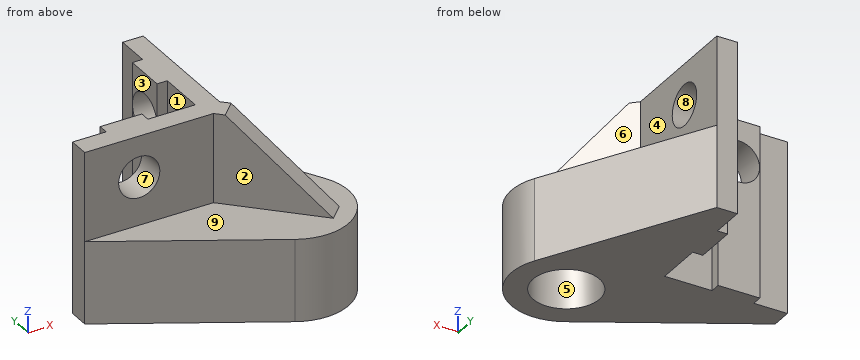
from build123d import *

# Parameters (mm, degrees)
BOSS_EXTRUDE1_DEPTH = 25
SKETCH2_R           = 3
CUT_EXTRUDE1_DEPTH  = 15
SKETCH3_R           = 3
CUT_EXTRUDE2_DEPTH  = 15
BOSS_EXTRUDE2_DEPTH = 12
BOSS_EXTRUDE4_DEPTH = 1.5
SKETCH6_R           = 4.85
CUT_EXTRUDE3_DEPTH  = 9


with BuildPart() as part:
    # Sketch1 → Boss-Extrude1 (new body)
    with BuildSketch(Plane.XY):
        Polygon((227.088719843, 62.282971172), (227.088719843, 57.379571172), (225.590119843, 57.379571172), (225.590119843, 51.299571172), (227.088719843, 51.299571172), (227.088719843, 44.429550862), (220.178702595, 44.429550862), (220.178702595, 45.917195068), (214.098687419, 45.917195068), (214.098687419, 44.429550862), (209.19527518, 44.429550862), (209.19527518, 41.429550862), (230.088719843, 41.429550862), (230.088719843, 62.282971172), align=None)
    extrude(amount=-BOSS_EXTRUDE1_DEPTH)

    # Sketch2 → Cut-Extrude1 (cut)
    with BuildSketch(Plane(origin=(230.088719843, 0, 0), x_dir=(0, 0, -1), z_dir=(1, 0, 0))):
        with Locations((6, 54.339571172)):
            Circle(SKETCH2_R)
    extrude(amount=-CUT_EXTRUDE1_DEPTH, mode=Mode.SUBTRACT)

    # Sketch3 → Cut-Extrude2 (cut)
    with BuildSketch(Plane.XZ.offset(-41.429550862)):
        with Locations((217.138695007, -6)):
            Circle(SKETCH3_R)
    extrude(amount=-CUT_EXTRUDE2_DEPTH, mode=Mode.SUBTRACT)

    # Sketch4 → Boss-Extrude2 (add)
    with BuildSketch(Plane(origin=(0, 0, -25), x_dir=(-1, 0, 0), z_dir=(0, 0, -1))):
        with BuildLine():
            Line((-230.088719843, 62.282971172), (-243.051733392, 39.368642422))
            ThreePointArc((-243.051733392, 39.368642422), (-241.747687926, 29.774811236), (-232.154834185, 28.463594817))
            Line((-232.154834185, 28.463594817), (-209.19527518, 41.429550862))
            Line((-209.19527518, 41.429550862), (-230.088719843, 41.429550862))
            Line((-230.088719843, 41.429550862), (-230.088719843, 62.282971172))
        make_face()
    extrude(amount=-BOSS_EXTRUDE2_DEPTH)

    # Sketch5 → Boss-Extrude4 (add, symmetric)
    with BuildSketch(Plane(origin=(135.717402312, 135.766641949, 0), x_dir=(0.707235019, -0.70697852, 0), z_dir=(-0.70697852, -0.707235019, 0))):
        Polygon((133.436997596, -13), (147.436997596, -13), (133.436997596, 0), (129.194356979, 0), (129.194356979, -13), align=None)
    extrude(amount=BOSS_EXTRUDE4_DEPTH, both=True)

    # Sketch6 → Cut-Extrude3 (cut)
    with BuildSketch(Plane(origin=(0, 0, -25), x_dir=(-1, 0, 0), z_dir=(0, 0, -1))):
        with Locations((-236.088719843, 35.429550862)):
            Circle(SKETCH6_R)
    extrude(amount=-CUT_EXTRUDE3_DEPTH, mode=Mode.SUBTRACT)


solid = part.part
Geometry check sheet. Reference: the model listing, model coordinates, mm. Face numbers are marked on the shaded views. A direction names the side the tool comes from. Give positions to 0.01 mm unless a question says otherwise; leave off trailing zeros. Order: outer loops, then holes, each group sorted by start corner. A loop starts at its lowest first (then second) coordinate and runs counter-clockwise, first axis right, second up. Notation, with made-up numbers: (38.25, 49.5) - (51.25, 49.5) arc R21 cw to (51.25, 83.5) - close; hole circle Ø10 at (58, 56.5). An arc over 180 degrees is marked (long way). Answer as a JSON object with one key per item and string values.
(1) Tool access check on the marked faces 1, 2, 3, 4 and 5. Record the directions out of +Z, -Z, +X, -X, +Y, -Y that give a thin tool (end or side, any length) a straight path to the whole face; none if there is none.
Report:
{"face 1": "+Z, -Z", "face 2": "+Z, -X, -Y", "face 3": "+Z, -Z, -X, +Y", "face 4": "+Z, +X, +Y", "face 5": "-Z"}
(2) Draft check along Z on the marked faces 6, 7, 8 and 9. Enter one of: released by +Z, released by -Z, zero draft, split by the parting line, or undercut.
Report:
{"face 6": "zero draft", "face 7": "undercut", "face 8": "undercut", "face 9": "released by +Z"}
(3) Depth check by flat-ended pin: pin 1 Ø5 at (x, z) = (218.5, -18) entering from -Y; pin 2 Ø0.7 at (y, z) = (45, -6.5) entering from -X; pin 3 Ø2 at (x, z) = (222.5, -17) entering from +Y. Enter the tip coordinate at first touch or a pass-through.
Report:
{"pin 1": "y = 34.76", "pin 2": "x = 214.1", "pin 3": "y = 44.43"}
(4) Cross-section at C-C (z = -11.25). Record the cut outline in (x, y).
Report:
{"outline": "(209.2, 41.43) - (227.97, 41.43) - (237.6, 31.8) - (239.72, 33.93) - (230.09, 43.55) - (230.09, 62.28) - (227.09, 62.28) - (227.09, 57.38) - (225.59, 57.38) - (225.59, 51.3) - (227.09, 51.3) - (227.09, 44.43) - (220.18, 44.43) - (220.18, 45.92) - (214.1, 45.92) - (214.1, 44.43) - (209.2, 44.43) - close"}
(5) Cross-section at D-D (y = 55.5). Record the cut outline in (x, z).
Report:
{"outline": "(225.59, -25) - (233.93, -25) - (233.93, -13) - (230.09, -13) - (230.09, -8.77) - (225.59, -8.77) - close; (225.59, -3.23) - (230.09, -3.23) - (230.09, 0) - (225.59, 0) - close"}
(6) Cross-section at B-B (z = -6). State how many separate pieces and enclosed holes the cut face has, then the cut area to 3 significant figures.
Report:
{"separate pieces": "3", "enclosed holes": "0", "area": "102 mm^2"}
(7) Material ranges on line 1 (Y direction, x = 228.5, z = -5.5); line 2 (Z direction, x = 232, y = 57); line 3 (Z direction, x = 228.5, y = 56.5), recorded low to high.
Report:
{"line 1": "40.9 to 51.38, 57.3 to 62.28", "line 2": "-25 to -13", "line 3": "-25 to -8.08, -3.92 to 0"}
(8) Cross-section at A-A (y = 52). Record the cut outline in (x, z), then the cut area to 3 significant figures.
Report:
{"outline": "(225.59, -25) - (235.91, -25) - (235.91, -13) - (230.09, -13) - (230.09, -7.88) - (225.59, -7.88) - close; (225.59, -4.12) - (230.09, -4.12) - (230.09, 0) - (225.59, 0) - close", "area": "165 mm^2"}
